from build123d import *

# Parameters (mm, degrees)
SKETCH1_R           = 3.55
SKETCH1_R_2         = 1.25
BOSS_EXTRUDE1_DEPTH = 2.3
BOSS_EXTRUDE2_START = 2.3
SKETCH1_3_R         = 3.55
SKETCH1_3_R_2       = 1.25
BOSS_EXTRUDE2_DEPTH = 1.85
BOSS_EXTRUDE3_START = 2.3
BOSS_EXTRUDE3_DEPTH = 9
CUT_EXTRUDE3_REACH  = 73.238
SKETCH2_W           = 7.938
SKETCH2_H           = 8.3
CUT_EXTRUDE4_REACH  = 73.092
SKETCH3_W           = 13.048
SKETCH3_H           = 6.12
CUT_EXTRUDE5_REACH  = 73.092
SKETCH4_W           = 12.28
SKETCH4_H           = 7.81
SKETCH5_R           = 1.6
BOSS_EXTRUDE4_DEPTH = 3
FILLET1_R           = 2


with BuildPart() as part:
    # Sketch1 → Boss-Extrude1 (new body)
    # profile 1 of 7: a face of its own
    with BuildSketch(Plane(origin=(0, 0, 0), x_dir=(1, 0, 0), z_dir=(0, 1, 0))):
        with BuildLine():
            ThreePointArc((-3.5, -3.556), (-1.433345448, 1.433345448), (3.556, 3.5))
            Line((3.556, 3.5), (42.304, 3.5))
            ThreePointArc((42.304, 3.5), (47.293345448, 1.433345448), (49.36, -3.556))
            Line((49.36, -3.556), (49.36, -39.344))
            ThreePointArc((49.36, -39.344), (47.293345448, -44.333345448), (42.304, -46.4))
            Line((42.304, -46.4), (3.556, -46.4))
            ThreePointArc((3.556, -46.4), (-1.433345448, -44.333345448), (-3.5, -39.344))
            Line((-3.5, -39.344), (-3.5, -3.556))
        make_face()
        with BuildLine():
            Line((-0.5, -3.556), (-0.5, -39.344))
            ThreePointArc((-0.5, -39.344), (0.687974896, -42.212025104), (3.556, -43.4))
            Line((3.556, -43.4), (42.304, -43.4))
            ThreePointArc((42.304, -43.4), (45.172025104, -42.212025104), (46.36, -39.344))
            Line((46.36, -39.344), (46.36, -3.556))
            ThreePointArc((46.36, -3.556), (45.172025104, -0.687974896), (42.304, 0.5))
            Line((42.304, 0.5), (3.556, 0.5))
            ThreePointArc((3.556, 0.5), (0.687974896, -0.687974896), (-0.5, -3.556))
        make_face(mode=Mode.SUBTRACT)
    # profile 2 of 7: a face of its own
    with BuildSketch(Plane(origin=(0, 0, 0), x_dir=(1, 0, 0), z_dir=(0, 1, 0))):
        with BuildLine():
            ThreePointArc((-0.5, -3.556), (0.687974896, -0.687974896), (3.556, 0.5))
            Line((3.556, 0.5), (42.304, 0.5))
            ThreePointArc((42.304, 0.5), (45.172025104, -0.687974896), (46.36, -3.556))
            Line((46.36, -3.556), (46.36, -39.344))
            ThreePointArc((46.36, -39.344), (45.172025104, -42.212025104), (42.304, -43.4))
            Line((42.304, -43.4), (3.556, -43.4))
            ThreePointArc((3.556, -43.4), (0.687974896, -42.212025104), (-0.5, -39.344))
            Line((-0.5, -39.344), (-0.5, -3.556))
        make_face()
        with BuildLine():
            Line((0, -3.556), (0, -39.344))
            ThreePointArc((0, -39.344), (1.041528286, -41.858471714), (3.556, -42.9))
            Line((3.556, -42.9), (42.304, -42.9))
            ThreePointArc((42.304, -42.9), (44.818471714, -41.858471714), (45.86, -39.344))
            Line((45.86, -39.344), (45.86, -3.556))
            ThreePointArc((45.86, -3.556), (44.818471714, -1.041528286), (42.304, 0))
            Line((42.304, 0), (3.556, 0))
            ThreePointArc((3.556, 0), (1.041528286, -1.041528286), (0, -3.556))
        make_face(mode=Mode.SUBTRACT)
    # profile 3 of 7: a face of its own
    with BuildSketch(Plane(origin=(0, 0, 0), x_dir=(1, 0, 0), z_dir=(0, 1, 0))):
        with BuildLine():
            ThreePointArc((0, -3.556), (1.041528286, -1.041528286), (3.556, 0))
            Line((3.556, 0), (42.304, 0))
            ThreePointArc((42.304, 0), (44.818471714, -1.041528286), (45.86, -3.556))
            Line((45.86, -3.556), (45.86, -39.344))
            ThreePointArc((45.86, -39.344), (44.818471714, -41.858471714), (42.304, -42.9))
            Line((42.304, -42.9), (3.556, -42.9))
            ThreePointArc((3.556, -42.9), (1.041528286, -41.858471714), (0, -39.344))
            Line((0, -39.344), (0, -3.556))
        make_face()
        with Locations((3.556, -39.344)):
            Circle(SKETCH1_R, mode=Mode.SUBTRACT)
        with Locations((42.304, -39.344)):
            Circle(SKETCH1_R, mode=Mode.SUBTRACT)
        with Locations((42.304, -3.556)):
            Circle(SKETCH1_R, mode=Mode.SUBTRACT)
        with Locations((3.556, -3.556)):
            Circle(SKETCH1_R, mode=Mode.SUBTRACT)
    # profile 4 of 7: a face of its own
    with BuildSketch(Plane(origin=(0, 0, 0), x_dir=(1, 0, 0), z_dir=(0, 1, 0))):
        with Locations((42.304, -39.344)):
            Circle(SKETCH1_R)
        with Locations(Location((42.304, -39.344, 0), (0, 0, 270))):
            Circle(SKETCH1_R_2, mode=Mode.SUBTRACT)
    # profile 5 of 7: a face of its own
    with BuildSketch(Plane(origin=(0, 0, 0), x_dir=(1, 0, 0), z_dir=(0, 1, 0))):
        with Locations((3.556, -39.344)):
            Circle(SKETCH1_R)
        with Locations(Location((3.556, -39.344, 0), (0, 0, 270))):
            Circle(SKETCH1_R_2, mode=Mode.SUBTRACT)
    # profile 6 of 7: a face of its own
    with BuildSketch(Plane(origin=(0, 0, 0), x_dir=(1, 0, 0), z_dir=(0, 1, 0))):
        with Locations((3.556, -3.556)):
            Circle(SKETCH1_R)
        with Locations(Location((3.556, -3.556, 0), (0, 0, 270))):
            Circle(SKETCH1_R_2, mode=Mode.SUBTRACT)
    # profile 7 of 7: a face of its own
    with BuildSketch(Plane(origin=(0, 0, 0), x_dir=(1, 0, 0), z_dir=(0, 1, 0))):
        with Locations((42.304, -3.556)):
            Circle(SKETCH1_R)
        with Locations(Location((42.304, -3.556, 0), (0, 0, 270))):
            Circle(SKETCH1_R_2, mode=Mode.SUBTRACT)
    extrude(amount=BOSS_EXTRUDE1_DEPTH)

    # Sketch1<3> → Boss-Extrude2 (add)
    # profile 1 of 4: a face of its own
    with BuildSketch(Plane(origin=(0, 0, 0), x_dir=(1, 0, 0), z_dir=(0, 1, 0)).offset(BOSS_EXTRUDE2_START)):
        with Locations(Location((3.556, -3.556, 0), (0, 0, 270))):
            Circle(SKETCH1_3_R)
        with Locations(Location((3.556, -3.556, 0), (0, 0, 270))):
            Circle(SKETCH1_3_R_2, mode=Mode.SUBTRACT)
    # profile 2 of 4: a face of its own
    with BuildSketch(Plane(origin=(0, 0, 0), x_dir=(1, 0, 0), z_dir=(0, 1, 0)).offset(BOSS_EXTRUDE2_START)):
        with Locations(Location((42.304, -3.556, 0), (0, 0, 270))):
            Circle(SKETCH1_3_R)
        with Locations(Location((42.304, -3.556, 0), (0, 0, 270))):
            Circle(SKETCH1_3_R_2, mode=Mode.SUBTRACT)
    # profile 3 of 4: a face of its own
    with BuildSketch(Plane(origin=(0, 0, 0), x_dir=(1, 0, 0), z_dir=(0, 1, 0)).offset(BOSS_EXTRUDE2_START)):
        with Locations(Location((42.304, -39.344, 0), (0, 0, 270))):
            Circle(SKETCH1_3_R)
        with Locations(Location((42.304, -39.344, 0), (0, 0, 270))):
            Circle(SKETCH1_3_R_2, mode=Mode.SUBTRACT)
    # profile 4 of 4: a face of its own
    with BuildSketch(Plane(origin=(0, 0, 0), x_dir=(1, 0, 0), z_dir=(0, 1, 0)).offset(BOSS_EXTRUDE2_START)):
        with Locations(Location((3.556, -39.344, 0), (0, 0, 270))):
            Circle(SKETCH1_3_R)
        with Locations(Location((3.556, -39.344, 0), (0, 0, 270))):
            Circle(SKETCH1_3_R_2, mode=Mode.SUBTRACT)
    extrude(amount=BOSS_EXTRUDE2_DEPTH)

    # Sketch1<4> → Boss-Extrude3 (add)
    with BuildSketch(Plane(origin=(0, 0, 0), x_dir=(1, 0, 0), z_dir=(0, 1, 0)).offset(BOSS_EXTRUDE3_START)):
        with BuildLine():
            ThreePointArc((-3.5, -3.556), (-1.433345448, 1.433345448), (3.556, 3.5))
            Line((3.556, 3.5), (42.304, 3.5))
            ThreePointArc((42.304, 3.5), (47.293345448, 1.433345448), (49.36, -3.556))
            Line((49.36, -3.556), (49.36, -39.344))
            ThreePointArc((49.36, -39.344), (47.293345448, -44.333345448), (42.304, -46.4))
            Line((42.304, -46.4), (3.556, -46.4))
            ThreePointArc((3.556, -46.4), (-1.433345448, -44.333345448), (-3.5, -39.344))
            Line((-3.5, -39.344), (-3.5, -3.556))
        make_face()
        with BuildLine():
            Line((-0.5, -3.556), (-0.5, -39.344))
            ThreePointArc((-0.5, -39.344), (0.687974896, -42.212025104), (3.556, -43.4))
            Line((3.556, -43.4), (42.304, -43.4))
            ThreePointArc((42.304, -43.4), (45.172025104, -42.212025104), (46.36, -39.344))
            Line((46.36, -39.344), (46.36, -3.556))
            ThreePointArc((46.36, -3.556), (45.172025104, -0.687974896), (42.304, 0.5))
            Line((42.304, 0.5), (3.556, 0.5))
            ThreePointArc((3.556, 0.5), (0.687974896, -0.687974896), (-0.5, -3.556))
        make_face(mode=Mode.SUBTRACT)
    extrude(amount=BOSS_EXTRUDE3_DEPTH)

    # Sketch2 → Cut-Extrude3 (cut, up to next)
    with BuildSketch(Plane(origin=(49.36, 0, 0), x_dir=(0, 0, -1), z_dir=(1, 0, 0)), mode=Mode.PRIVATE) as cut_extrude3_sk1:
        with Locations((-26.725, 7.15)):
            Rectangle(SKETCH2_W, SKETCH2_H)
    cut_extrude3_tool1 = extrude(cut_extrude3_sk1.sketch, amount=-CUT_EXTRUDE3_REACH, mode=Mode.PRIVATE) & part.part
    add(cut_extrude3_tool1.solids().sort_by_distance((49.36, 7.15, 26.725))[0], mode=Mode.SUBTRACT)

    # Sketch3 → Cut-Extrude4 (cut, up to next)
    with BuildSketch(Plane.XY.offset(46.4), mode=Mode.PRIVATE) as cut_extrude4_sk1:
        with Locations((13.58, 8.24)):
            Rectangle(SKETCH3_W, SKETCH3_H)
    cut_extrude4_tool1 = extrude(cut_extrude4_sk1.sketch, amount=-CUT_EXTRUDE4_REACH, mode=Mode.PRIVATE) & part.part
    add(cut_extrude4_tool1.solids().sort_by_distance((13.58, 8.24, 46.4))[0], mode=Mode.SUBTRACT)

    # Sketch4 → Cut-Extrude5 (cut, up to next)
    with BuildSketch(Plane.XY.offset(46.4), mode=Mode.PRIVATE) as cut_extrude5_sk1:
        with Locations((25.394, 7.395)):
            Rectangle(SKETCH4_W, SKETCH4_H)
    cut_extrude5_tool1 = extrude(cut_extrude5_sk1.sketch, amount=-CUT_EXTRUDE5_REACH, mode=Mode.PRIVATE) & part.part
    add(cut_extrude5_tool1.solids().sort_by_distance((25.394, 7.395, 46.4))[0], mode=Mode.SUBTRACT)

    # Sketch5 → Boss-Extrude4 (add)
    # profile 1 of 2: a face of its own
    with BuildSketch(Plane.XZ):
        with BuildLine():
            Line((-3.5, 16.45), (-10, 16.45))
            ThreePointArc((-10, 16.45), (-12.474873734, 17.475126266), (-13.5, 19.95))
            Line((-13.5, 19.95), (-13.5, 22.95))
            ThreePointArc((-13.5, 22.95), (-12.474873734, 25.424873734), (-10, 26.45))
            Line((-10, 26.45), (-3.5, 26.45))
            Line((-3.5, 26.45), (-3.5, 16.45))
        make_face()
        with Locations(Location((-8.5, 21.45, 0), (0, 0, 270))):
            Circle(SKETCH5_R, mode=Mode.SUBTRACT)
    # profile 2 of 2: a face of its own
    with BuildSketch(Plane.XZ):
        with BuildLine():
            Line((49.36, 16.45), (55.86, 16.45))
            ThreePointArc((55.86, 16.45), (58.334873734, 17.475126266), (59.36, 19.95))
            Line((59.36, 19.95), (59.36, 22.95))
            ThreePointArc((59.36, 22.95), (58.334873734, 25.424873734), (55.86, 26.45))
            Line((55.86, 26.45), (49.36, 26.45))
            Line((49.36, 26.45), (49.36, 16.45))
        make_face()
        with Locations(Location((54.36, 21.45, 0), (0, 0, 270))):
            Circle(SKETCH5_R, mode=Mode.SUBTRACT)
    extrude(amount=-BOSS_EXTRUDE4_DEPTH)

    # Fillet1
    fillet1_edges = [part.edges().sort_by_distance(p)[0] for p in [
        (49.36, 3, 28.572),
        (-3.5, 3, 21.45),
        (-3.5, 1.5, 26.45),
        (-6.75, 3, 16.45),
        (-3.5, 1.5, 16.45),
        (-12.474873734, 3, 17.475126266),
        (-13.5, 3, 21.45),
        (-12.474873734, 3, 25.424873734),
        (-6.75, 3, 26.45),
        (49.36, 3, 19.603),
        (49.36, 1.5, 16.45),
        (52.61, 3, 26.45),
        (49.36, 1.5, 26.45),
        (58.334873734, 3, 25.424873734),
        (59.36, 3, 21.45),
        (58.334873734, 3, 17.475126266),
        (52.61, 3, 16.45),
    ]]
    fillet(fillet1_edges, radius=FILLET1_R)


solid = part.part
Geometry: final body of the model. Coordinates: model frame, mm. A direction names the side the tool comes from. Round coordinates to 2 decimals unless told otherwise and drop trailing zeros. Loops run counter-clockwise (first coordinate to the right, second up) from the corner with the lowest first, then second, coordinate; pieces in that order, holes last. Notation, with made-up numbers: M -17.5,53 L -4.5,53 A26 ccw -4.5,89 Z; hole C -26.5,14 d1. An arc over 180 degrees is marked long. Put each result on its own line as item: value. Start each with the question number.
(1) Section query A-A (z = 21.45). Return loops of the section in (x, y).
(2) Draft query along X for faces 5 (the face through (49.96, 0.51, 27.02)), 6 (the face through (-7, 3, 20)), 7 (the face through (3.931, 2.046, 40.536)). Return one class per face: +X half, -X half, draft (parallel to the pull), parting line (faces both ways), or undercut.
(3) Set-up query: faces 1 (the face through (-7.78, 2.43, 17.05)), 2 (the face through (51, 3, 23)), 3 (the face through (58.31, 0.49, 17.45)), 4 (the face through (7.076, 3.212, 3.094)). Return all of +Z, -Z, +X, -X, +Y, -Y with unobstructed straight access to the full face (end or side cutting, diameter ignored); none if empty.
(4) Section query D-D (x = 32.5). Return loops of the section in (y, z).
(5) Material intervals for line 1 along X through (y, z) = (3.5, 34); line 2 along Z through (x, y) = (33.5, 6); line 3 along X through (y, z) = (0.75, 4.5), sorted ascending. Write a range as [from, to].
(6) Section query C-C (x = -8.5). Return loops of the section in (y, z), then the cut area to 3 significant figures.
(7) Contact query for flat-ended pins moving along their axis: pin 1 Ø3 at (y, z) = (2, 31.5) entering from -X; pin 2 Ø2 at (x, z) = (42, 2.5) entering from +Y; pin 3 Ø2.5 at (x, z) = (23.5, 45.5) entering from +Y. Output: stop coordinate, or through.
(8) Section query B-B (y = 8.75). Return loops of the section in (x, z), then the cut area to 3 significant figures.
Findings below:
1. outline: M -13.5,0 L -10.1,0 L -10.1,3 L -11.5,3 A2 ccw -13.5,1 Z; M -6.9,0 L 52.76,0 L 52.76,3 L 51.36,3 A2 cw 49.36,5 L 49.36,11.3 L 46.36,11.3 L 46.36,2.3 L -0.5,2.3 L -0.5,11.3 L -3.5,11.3 L -3.5,5 A2 cw -5.5,3 L -6.9,3 Z; M 55.96,0 L 59.36,0 L 59.36,1 A2 ccw 57.36,3 L 55.96,3 Z
2. face 5: +X half
2. face 6: draft
2. face 7: undercut
3. face 1: -Z, -X, +Y
3. face 2: +X, +Y
3. face 3: -Z, +X, +Y, -Y
3. face 4: +Y
4. outline: M 0,-3.5 L 11.3,-3.5 L 11.3,-0.5 L 2.3,-0.5 L 2.3,43.4 L 11.3,43.4 L 11.3,46.4 L 0,46.4 Z
5. line 1: x = [-3.5, -0.5], [46.36, 49.36]
5. line 2: z = [-3.5, -0.5], [43.4, 46.4]
5. line 3: x = [-3.5, 2.74], [4.38, 41.48], [43.12, 49.36]
6. outline: M 0,16.45 L 1,16.45 A2 ccw 3,18.45 L 3,19.85 L 0,19.85 Z; M 0,23.05 L 3,23.05 L 3,24.45 A2 ccw 1,26.45 L 0,26.45 Z
6. area: 18.7 mm2
7. pin 1: stops at x = -3.5
7. pin 2: stops at y = 4.15
7. pin 3: stops at y = 3.49
8. outline: M -3.5,3.56 A7.06 ccw 3.56,-3.5 L 42.3,-3.5 A7.06 ccw 49.36,3.56 L 49.36,22.76 L 46.36,22.76 L 46.36,3.56 A4.06 cw 42.3,-0.5 L 3.56,-0.5 A4.06 cw -0.5,3.56 L -0.5,39.34 A4.06 cw 3.56,43.4 L 7.06,43.4 L 7.06,46.4 L 3.56,46.4 A7.06 ccw -3.5,39.34 Z; M 31.53,43.4 L 42.3,43.4 A4.06 cw 46.36,39.34 L 46.36,30.69 L 49.36,30.69 L 49.36,39.34 A7.06 ccw 42.3,46.4 L 31.53,46.4 Z
8. area: 455 mm2
